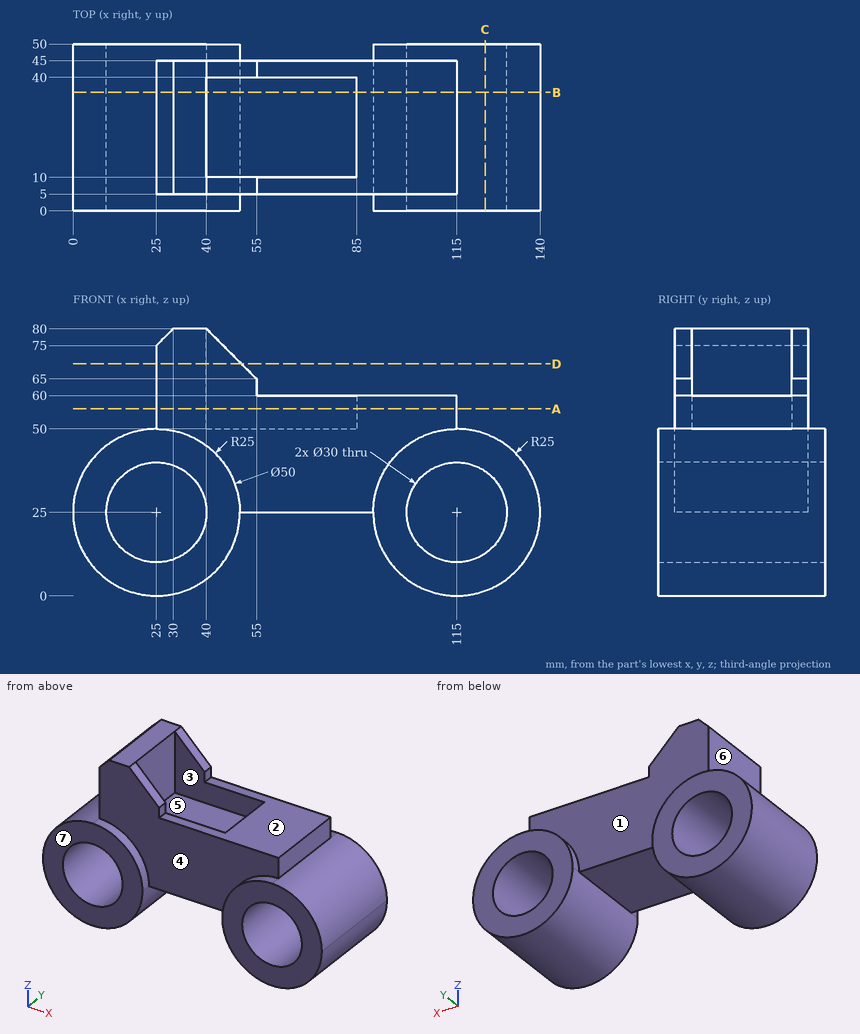
Check sheet for the drawn part. Datum: minimum x, y, z corner. Units: mm. A direction names the side the tool comes from. Coordinates: 2 decimals unless noted, no trailing zeros. Order: outer loops, then holes, each group sorted by start corner. A loop starts at its lowest first (then second) coordinate and runs counter-clockwise, first axis right, second up. Notation, with made-up numbers: M -9.75,14 L 14.25,14 A20 ccw 14.25,31 Z; hole C 52,53 d10. An arc over 180 degrees is marked long. One line per question, with ' | ' between items. Start each with the question number.
Item 1: Cross-section at B-B on y = 35.5. Enter the section's corners in (x, z).
Item 2: Material ranges on L1, parallel to X at y = 6.5, z = 24; L2, parallel to Z at x = 115.5, y = 42 (3 decimals); L3, parallel to X at y = 17, z = 32, recorded low to high. Write a range as [from, to].
Item 3: Draft check along X on the marked faces 5, 6 and 7. Enter one of: pulls with the +X half, pulls with the -X half, needs draft (parallel to the pull), parting line crosses it, or undercut.
Item 4: Cross-section at C-C on x = 123.5. Enter the section's corners in (y, z), then the cut area to 3 significant figures.
Item 5: Cross-section at A-A on z = 56. Enter the section's corners in (x, y).
Item 6: Gauge pin test, flat ends, axial feed: pin 1 (4 mm diameter, centred on x = 106.5, y = 8.5, fed in from +Z); pin 2 (12 mm diameter, centred on x = 54, z = 51.5, fed in from -Y); pin 3 (1.5 mm diameter, centred on x = 73.5, y = 34.5, fed in from +Z). Record the tip position at first contact, or that the pin passes through.
Item 7: Cross-section at D-D on z = 69.5. Enter the section's corners in (x, y), then the cut area to 3 significant figures.
Item 8: Set-up check for the marked faces 1, 2, 3 and 4: record each of +Z, -Z, +X, -X, +Y, -Y from which the full face is reachable in a straight line by a thin tool's end or side.
Findings:
1) outline: M 25,50 A25 ccw long 50,25 L 90,25 A25 ccw long 115,50 L 115,60 L 85,60 L 85,50 L 40,50 L 40,80 L 30,80 L 25,75 Z; hole C 25,25 d30; hole C 115,25 d30
2) L1: x = [0.02, 10.03], [39.97, 49.98], [90.02, 100.03], [129.97, 139.98] | L2: z = [0.005, 10.008], [39.992, 49.995] | L3: x = [1, 11.73], [38.27, 101.73], [128.27, 139]
3) face 5: undercut | face 6: pulls with the -X half | face 7: needs draft
4) outline: M 0,1.49 L 50,1.49 L 50,12.64 L 0,12.64 Z; M 0,37.36 L 50,37.36 L 50,48.51 L 0,48.51 Z | area: 1,120 mm²
5) outline: M 25,5 L 115,5 L 115,45 L 25,45 Z; hole M 40,10 L 85,10 L 85,40 L 40,40 Z
6) pin 1: stops at z = 60 | pin 2: stops at y = 5 | pin 3: stops at z = 50
7) outline: M 25,5 L 50.5,5 L 50.5,10 L 40,10 L 40,40 L 50.5,40 L 50.5,45 L 25,45 Z | area: 705 mm²
8) face 1: +Z, +Y | face 2: +Z, +X, +Y, -Y | face 3: +Z | face 4: +Z, -Y
